Here's how the part is built. I have some questions about the finished solid (model axes, mm). A direction names the side the tool comes from. Round coordinates to 2 decimals unless told otherwise and drop trailing zeros. Write each loop counter-clockwise with the first axis right and the second up, starting at its lowest first coordinate (ties: lowest second). Pieces come first, ordered by that corner, then holes. Notation, with made-up numbers: M 9,36 L 17,36 A18 ccw 17,58 Z; hole C -7.5,86.25 d5. An arc over 180 degrees is marked long. Write item = value, one per line. Start each with the question number.
(1) On a 3-axis mill with a long thin cutter (end or side, diameter ignored), from which of +Z, -Z, +X, -X, +Y, -Y can I reach the whole of each face in a straight line? I mean faces 4 (the flat face through (9, 187, -10.5)), 5 (the flat face through (10, 98, -12)), 6 (the flat face through (6, 189, -8.082)). Say none if no direction works.
(2) Will these pins go through, and if not, where does the flat tip stop? pin 1 Ø5 at (x, z) = (5, -6) entering from -Y; pin 2 Ø2 at (x, z) = (12.5, -16.5) entering from +Y; pin 3 Ø3 at (y, z) = (43.5, -19) entering from +X.
(3) I want a section at B-B (y = 187.5). List the corners of the cut face in (x, z) for me.
(4) If we mould it in two halves opening along Y, with no side actions, what happens to faces 1 (the flat face through (6, 189, -5.082)), 2 (the flat face through (14, 99, -1)), 3 (the cylindrical face through (7.1, 197.15, -3.01))? For each: released by +Y, released by -Y, zero draft, split by the parting line, or undercut.
(5) I want a section at A-A (y = 12.5). List the corners of the cut face in (x, z) for me, and give its area (3 significant figures).
(6) I need wall thicknesses on line 1 along Y through (x, z) = (4.25, -12.5); line 2 along Z through (x, y) = (2.5, 189); line 3 along X through (y, z) = (187.5, -4). Which ranges of each line are inside material? Lowest first, please.
```python
from build123d import *

# Parameters (mm, degrees)
CROQUIS1_W              = 14
CROQUIS1_H              = 25
SALIENTE_EXTRUIR1_DEPTH = 200
REDONDEO1_R             = 10
REDONDEO2_R             = 10
CROQUIS2_R              = 8.6
CORTAR_EXTRUIR1_DEPTH   = 28
CROQUIS14_R             = 9.913044
SALIENTE_EXTRUIR2_DEPTH = 14
CROQUIS12_R             = 2
CORTAR_EXTRUIR7_DEPTH   = 203.042074826
CROQUIS15_W             = 3
CROQUIS15_H             = 5.6
CORTAR_EXTRUIR9_DEPTH   = 8
CROQUIS16_W             = 17
CROQUIS16_H             = 145
CORTAR_EXTRUIR10_DEPTH  = 4
CROQUIS17_W             = 17
CROQUIS17_H             = 145
CORTAR_EXTRUIR11_DEPTH  = 4
REDONDEO5_R             = 2
REDONDEO6_R             = 2
CROQUIS18_W             = 1
CROQUIS18_H             = 1
CORTAR_EXTRUIR12_DEPTH  = 203.042074845
REDONDEO9_R             = 10
REDONDEO10_R            = 10


with BuildPart() as part:
    # Croquis1 → Saliente-Extruir1 (new body)
    with BuildSketch(Plane(origin=(0, 0, 0), x_dir=(1, 0, 0), z_dir=(0, 1, 0))):
        with Locations((7, 12.5)):
            Rectangle(CROQUIS1_W, CROQUIS1_H)
    extrude(amount=SALIENTE_EXTRUIR1_DEPTH)

    # Redondeo1
    redondeo1_edges = [part.edges().sort_by_distance(p)[0] for p in [
        (7, 0, -25),
    ]]
    fillet(redondeo1_edges, radius=REDONDEO1_R)

    # Redondeo2
    redondeo2_edges = [part.edges().sort_by_distance(p)[0] for p in [
        (7, 0, 0),
    ]]
    fillet(redondeo2_edges, radius=REDONDEO2_R)

    # Croquis2 → Cortar-Extruir1 (cut)
    with BuildSketch(Plane(origin=(14, 0, 0), x_dir=(0, 0, -1), z_dir=(1, 0, 0))):
        with Locations((12.5, 12.5)):
            Circle(CROQUIS2_R)
        with BuildLine():
            Line((10.5, 185.263932023), (10.5, 189.736067977))
            ThreePointArc((10.5, 189.736067977), (15.5, 187.5), (10.5, 185.263932023))
        make_face()
    extrude(amount=-CORTAR_EXTRUIR1_DEPTH, mode=Mode.SUBTRACT)

    # Croquis14 → Saliente-Extruir2 (add)
    with BuildSketch(Plane(origin=(14, 0, 0), x_dir=(0, 0, -1), z_dir=(1, 0, 0))):
        with Locations((12.5, 187.5)):
            Circle(CROQUIS14_R)
        with BuildLine():
            Line((10.5, 185.263932023), (10.5, 189.736067977))
            ThreePointArc((10.5, 189.736067977), (15.5, 187.5), (10.5, 185.263932023))
        make_face(mode=Mode.SUBTRACT)
    extrude(amount=-SALIENTE_EXTRUIR2_DEPTH)

    # Croquis12 → Cortar-Extruir7 (cut, through all)
    with BuildSketch(Plane(origin=(0, 0, -25), x_dir=(-1, 0, 0), z_dir=(0, 0, -1))):
        with Locations((-4, 187.5)):
            Circle(CROQUIS12_R)
    extrude(amount=-CORTAR_EXTRUIR7_DEPTH, mode=Mode.SUBTRACT)

    # Croquis15 → Cortar-Extruir9 (cut)
    with BuildSketch(Plane.ZY):
        with Locations((-6.582205818, 187.5)):
            Rectangle(CROQUIS15_W, CROQUIS15_H)
    extrude(amount=-CORTAR_EXTRUIR9_DEPTH, mode=Mode.SUBTRACT)

    # Croquis16 → Cortar-Extruir10 (cut)
    with BuildSketch(Plane.ZY):
        with Locations((-12.5, 97.5)):
            Rectangle(CROQUIS16_W, CROQUIS16_H)
    extrude(amount=-CORTAR_EXTRUIR10_DEPTH, mode=Mode.SUBTRACT)

    # Croquis17 → Cortar-Extruir11 (cut)
    with BuildSketch(Plane(origin=(14, 0, 0), x_dir=(0, 0, -1), z_dir=(1, 0, 0))):
        with Locations((12.5, 97.5)):
            Rectangle(CROQUIS17_W, CROQUIS17_H)
    extrude(amount=-CORTAR_EXTRUIR11_DEPTH, mode=Mode.SUBTRACT)

    # Redondeo5
    redondeo5_edges = [part.edges().sort_by_distance(p)[0] for p in [
        (4, 97.5, -21),
        (4, 170, -12.5),
        (4, 97.5, -4),
        (4, 25, -12.5),
    ]]
    fillet(redondeo5_edges, radius=REDONDEO5_R)

    # Redondeo6
    redondeo6_edges = [part.edges().sort_by_distance(p)[0] for p in [
        (10, 97.5, -21),
        (10, 25, -12.5),
        (10, 97.5, -4),
        (10, 170, -12.5),
    ]]
    fillet(redondeo6_edges, radius=REDONDEO6_R)

    # Croquis18 → Cortar-Extruir12 (cut, through all)
    with BuildSketch(Plane(origin=(14, 0, 0), x_dir=(0, 0, -1), z_dir=(1, 0, 0))):
        with Locations((12.5, 199.5)):
            Rectangle(CROQUIS18_W, CROQUIS18_H)
    extrude(amount=-CORTAR_EXTRUIR12_DEPTH, mode=Mode.SUBTRACT)

    # Redondeo9
    redondeo9_edges = [part.edges().sort_by_distance(p)[0] for p in [
        (7, 200, 0),
    ]]
    fillet(redondeo9_edges, radius=REDONDEO9_R)

    # Redondeo10
    redondeo10_edges = [part.edges().sort_by_distance(p)[0] for p in [
        (7, 200, -25),
    ]]
    fillet(redondeo10_edges, radius=REDONDEO10_R)


solid = part.part
```
Returned:
q1.face_4 = +X, -X
q1.face_5 = +X
q1.face_6 = -X
q2.pin_1 = 0.11
q2.pin_2 = 199.99
q2.pin_3 = 10.68
q3.outline = M 0,-25 L 2,-25 L 2,-15.5 L 0,-15.5 Z; M 0,-10.5 L 2,-10.5 L 2,-8.08 L 0,-8.08 Z; M 0,-5.08 L 2,-5.08 L 2,0 L 0,0 Z; M 6,-25 L 14,-25 L 14,-15.5 L 6,-15.5 Z; M 6,-10.5 L 14,-10.5 L 14,0 L 6,0 L 6,-5.08 L 8,-5.08 L 8,-8.08 L 6,-8.08 Z
q4.face_1 = undercut
q4.face_2 = zero draft
q4.face_3 = released by +Y
q5.outline = M 0,-25 L 14,-25 L 14,-21.1 L 0,-21.1 Z; M 0,-3.9 L 14,-3.9 L 14,0 L 0,0 Z
q5.area = 109 mm²
q6.line_1 = 0 to 3.9, 21.1 to 184.5, 190.5 to 199
q6.line_2 = -25 to -15.1, -10.5 to -8.08, -5.08 to 0
q6.line_3 = 0 to 2, 6 to 14
